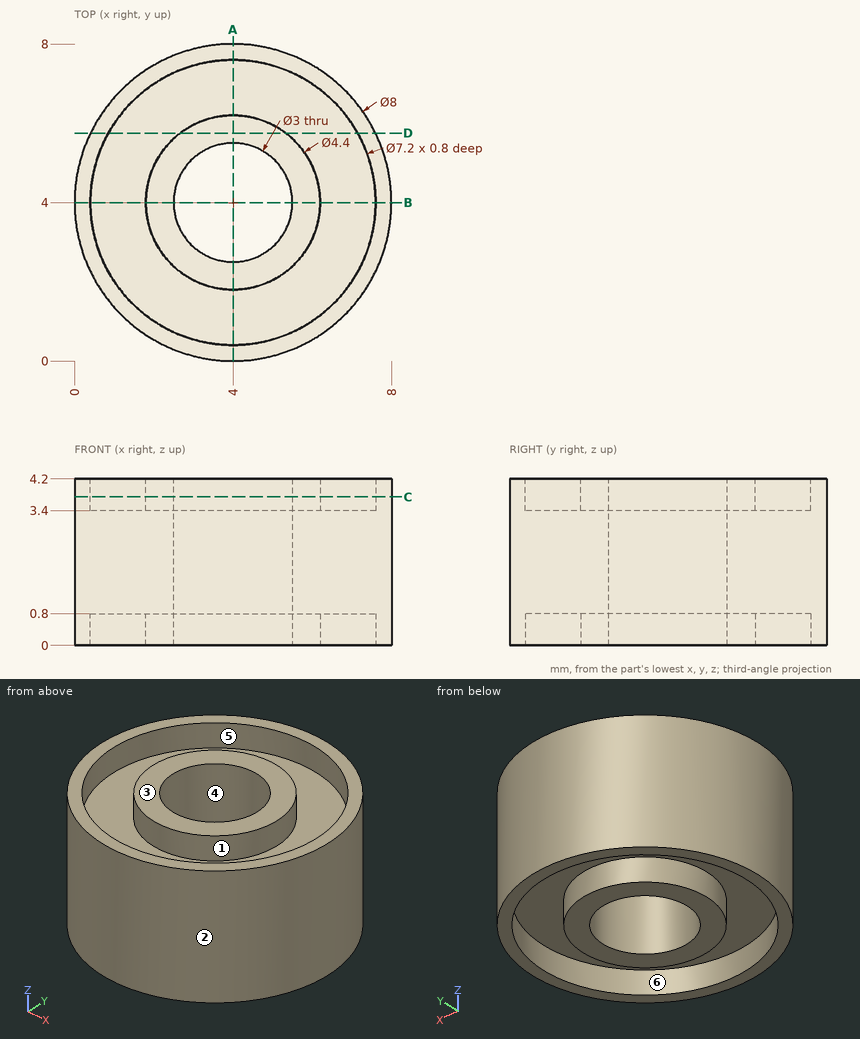
The figure shows three views and two pictorial views of one solid part (mm, origin at its lowest corner). Answer the questions. A direction names the side the tool comes from. Give positions to 0.01 mm unless a question says otherwise; leave off trailing zeros. Write each loop counter-clockwise with the first axis right and the second up, starting at its lowest first coordinate (ties: lowest second). Pieces come first, ordered by that corner, then holes. Notation, with made-up numbers: (36, 46.25) - (43, 46.25) arc R32 ccw to (43, 79.25) - close; hole circle Ø7 at (36.5, 36.5). An arc over 180 degrees is marked (long way). Use one line per item in the form item = value. Start each with the question number.
1) Flat-ended cylindrical pins translate along their axes: pin 1 Ø4.5 at (x, y) = (4, 4) entering from -Z; pin 2 Ø2.5 at (x, y) = (4, 4) entering from +Z; pin 3 Ø1.5 at (y, z) = (2.5, 3.5) entering from +X. Find the tip coordinate at first contact, or state that the pin passes through.
2) Consider line 1 along Y through (x, z) = (4, 0.5); line 2 along X through (y, z) = (3.75, 3.5); line 3 along Y through (x, z) = (4, 2.8). Determine where each line is inside the solid, lowest interval first. Write a range as from..to.
3) Find section C-C on z = 3.75. Determine the outline of the cut face in (x, y).
4) Find section D-D on y = 5.75. Determine the outline of the cut face in (x, z).
5) A tool of negligible diameter and unlimited length cuts with its end or side. For the marked faces 4, 5 and 6, from which of +Z, -Z, +X, -X, +Y, -Y can it reach the whole face along a straight path? Write none if from no direction.
6) Find section A-A on x = 4. Determine the outline of the cut face in (y, z), plus the area to 3 significant figures.
7) The mould has two halves that part along Y. Classify the marked faces 1, 2 and 3: pulls with the +Y half, pulls with the -Y half, needs draft (parallel to the pull), parting line crosses it, or undercut.
Geometry results:
q1.pin_1 = 0
q1.pin_2 = through
q1.pin_3 = 7.93
q2.line_1 = 0..0.4, 1.8..2.5, 5.5..6.2, 7.6..8
q2.line_2 = 0.01..0.41, 1.81..2.52, 5.48..6.19, 7.59..7.99
q2.line_3 = 0..2.5, 5.5..8
q3.outline = circle Ø8 at (4, 4); circle Ø4.4 at (4, 4); hole circle Ø7.2 at (4, 4); hole circle Ø3 at (4, 4)
q4.outline = (0.4, 0) - (0.85, 0) - (0.85, 0.8) - (2.67, 0.8) - (2.67, 0) - (5.33, 0) - (5.33, 0.8) - (7.15, 0.8) - (7.15, 0) - (7.6, 0) - (7.6, 4.2) - (7.15, 4.2) - (7.15, 3.4) - (5.33, 3.4) - (5.33, 4.2) - (2.67, 4.2) - (2.67, 3.4) - (0.85, 3.4) - (0.85, 4.2) - (0.4, 4.2) - close
q5.face_4 = +Z, -Z
q5.face_5 = +Z
q5.face_6 = -Z
q6.outline = (0, 0) - (0.4, 0) - (0.4, 0.8) - (1.8, 0.8) - (1.8, 0) - (2.5, 0) - (2.5, 4.2) - (1.8, 4.2) - (1.8, 3.4) - (0.4, 3.4) - (0.4, 4.2) - (0, 4.2) - close; (5.5, 0) - (6.2, 0) - (6.2, 0.8) - (7.6, 0.8) - (7.6, 0) - (8, 0) - (8, 4.2) - (7.6, 4.2) - (7.6, 3.4) - (6.2, 3.4) - (6.2, 4.2) - (5.5, 4.2) - close
q6.area = 16.5 mm2
q7.face_1 = undercut
q7.face_2 = parting line crosses it
q7.face_3 = needs draft
